Work out the finished part from the listing and answer in its coordinate system (mm). A direction names the side the tool comes from. Round coordinates to 2 decimals unless told otherwise and drop trailing zeros. Loops run counter-clockwise (first coordinate to the right, second up) from the corner with the lowest first, then second, coordinate; pieces in that order, holes last. Notation, with made-up numbers: (-13.75, 7) -> (16.25, 7) arc R13 cw to (16.25, 12) -> close; hole circle Ø3 at (-38.5, 38.5). An arc over 180 degrees is marked (long way). Write item = value, one per line. Start each with the question number.
```python
from build123d import *

# Parameters (mm, degrees)
F0_R     = 2.25
F0_R_2   = 1.5
F1_DEPTH = 2


with BuildPart() as f1:
    # F0 (on Top) → F1 (new body, symmetric)
    with BuildSketch(Plane.XY):
        with BuildLine():
            Line((46.25, 11), (57.25, 11))
            ThreePointArc((57.25, 11), (58.664214, 11.585786), (59.25, 13))
            Line((59.25, 13), (59.25, 18.5))
            ThreePointArc((59.25, 18.5), (58.634924, 19.984924), (57.15, 20.6))
            Line((57.15, 20.6), (53.15, 20.6))
            ThreePointArc((53.15, 20.6), (51.735786, 21.185786), (51.15, 22.6))
            Line((51.15, 22.6), (51.15, 32.5))
            ThreePointArc((51.15, 32.5), (50.564214, 33.914214), (49.15, 34.5))
            Line((49.15, 34.5), (-46.25, 34.5))
            ThreePointArc((-46.25, 34.5), (-47.664214, 33.914214), (-48.25, 32.5))
            Line((-48.25, 32.5), (-48.25, 31.5))
            ThreePointArc((-48.25, 31.5), (-48.835786, 30.085786), (-50.25, 29.5))
            Line((-50.25, 29.5), (-54.25, 29.5))
            ThreePointArc((-54.25, 29.5), (-55.664214, 28.914214), (-56.25, 27.5))
            Line((-56.25, 27.5), (-56.25, 24.5))
            ThreePointArc((-56.25, 24.5), (-55.664214, 23.085786), (-54.25, 22.5))
            Line((-54.25, 22.5), (-43.25, 22.5))
            ThreePointArc((-43.25, 22.5), (-41.835786, 23.085786), (-41.25, 24.5))
            Line((-41.25, 24.5), (-41.25, 27.5))
            Line((-41.25, 27.5), (42.25, 27.5))
            ThreePointArc((42.25, 27.5), (43.664214, 26.914214), (44.25, 25.5))
            Line((44.25, 25.5), (44.25, 13))
            ThreePointArc((44.25, 13), (44.835786, 11.585786), (46.25, 11))
        make_face()
        with Locations((55.15, 15.8)):
            Circle(F0_R, mode=Mode.SUBTRACT)
        with Locations((-52.25, 26)):
            Circle(F0_R, mode=Mode.SUBTRACT)
        with Locations((-24.85, 31)):
            Circle(F0_R_2, mode=Mode.SUBTRACT)
        with Locations((-2.85, 31)):
            Circle(F0_R_2, mode=Mode.SUBTRACT)
        with Locations((5.15, 31)):
            Circle(F0_R_2, mode=Mode.SUBTRACT)
        with Locations((27.55, 31)):
            Circle(F0_R_2, mode=Mode.SUBTRACT)
    extrude(amount=F1_DEPTH, both=True)


solid = f1.part
```
Item 1: Section A-A (x = 55.15) is taken. Determine the outline of the cut face in (y, z).
Item 2: Section D-D (x = -27.5) is taken. Determine the outline of the cut face in (y, z).
Item 3: A tool of negligible diameter and unlimited length cuts with its end or side. For faces 1 (the flat face through (52, 11, 0)), 2 (the cylindrical face through (43.65, 26.93, 0.03)), from which of +Z, -Z, +X, -X, +Y, -Y can it reach the whole face along a straight path? Write none if from no direction.
Item 4: The mould has two halves that part along X. Classify faces 3 (the flat face through (-41.25, 26, 0)), 4 (the flat face through (-49, 22.5, 0)), 5 (the flat face through (-56.25, 26, 0)): pulls with the +X half, pulls with the -X half, needs draft (parallel to the pull), parting line crosses it, or undercut.
Item 5: Section C-C (z = -0.55) is taken. Count the separate pieces of the cut face and the enclosed holes in it, then the cut area to 3 significant figures.
Item 6: Find the intervals of material crossed by line 1 along X through (y, z) = (25, -1.55); line 2 along Y through (x, z) = (17, 1.5); line 3 along Y through (x, z) = (-2.85, 0.75), in increasing order. Write a range as [from, to].
Item 7: Section B-B (y = 15.8) is taken. Determine the outline of the cut face in (x, z), then the cut area to 3 significant figures.
Item 8: Flat-ended cylindrical pins translate along their axes: pin 1 (0.5 mm diameter, centred on y = 32, z = -0.5, fed in from -X); pin 2 (1.2 mm diameter, centred on y = 26.5, z = -1, fed in from +X); pin 3 (1.2 mm diameter, centred on x = 55, z = 0, fed in from +Y); pin 4 (4 mm diameter, centred on x = -52.25, y = 26, fed in from -Z). Find the tip coordinate at first contact, or state that the pin passes through.
Worked answers:
q1.outline = (11, -2) -> (13.55, -2) -> (13.55, 2) -> (11, 2) -> close; (18.05, -2) -> (20.6, -2) -> (20.6, 2) -> (18.05, 2) -> close
q2.outline = (27.5, -2) -> (34.5, -2) -> (34.5, 2) -> (27.5, 2) -> close
q3.face_1 = +Z, -Z, +X, -X, -Y
q3.face_2 = +Z, -Z, -Y
q4.face_3 = undercut
q4.face_4 = needs draft
q4.face_5 = pulls with the -X half
q5.separate_pieces = 1
q5.enclosed_holes = 6
q5.area = 914 mm2
q6.line_1 = [-56.25, -54.27], [-50.23, -41.25], [44.25, 51.15]
q6.line_2 = [27.5, 34.5]
q6.line_3 = [27.5, 29.5], [32.5, 34.5]
q7.outline = (44.25, -2) -> (52.9, -2) -> (52.9, 2) -> (44.25, 2) -> close; (57.4, -2) -> (59.25, -2) -> (59.25, 2) -> (57.4, 2) -> close
q7.area = 42.0 mm2
q8.pin_1 = -48.25
q8.pin_2 = 51.15
q8.pin_3 = 20.6
q8.pin_4 = through
